Could you check a few things on this model? Use its own coordinates, in mm. A direction names the side the tool comes from. Round coordinates to 2 decimals unless told otherwise and drop trailing zeros. Loops run counter-clockwise (first coordinate to the right, second up) from the corner with the lowest first, then second, coordinate; pieces in that order, holes last. Notation, with made-up numbers: M 15,-28.75 L 58,-28.75 A13 ccw 58,-22.75 Z; hole C 45,88 d3. An arc over 180 degrees is marked long. Answer in a Markdown table with one row per item.
```python
from build123d import *

# Parameters (mm, degrees)
SKETCH1_R           = 14.642304845
BOSS_EXTRUDE1_DEPTH = 2.5
BOSS_EXTRUDE2_DEPTH = 2.5
CUT_EXTRUDE1_REACH  = 22.858
SKETCH3_R           = 2.1
SKETCH4_R           = 4.25
BOSS_EXTRUDE3_DEPTH = 1.75
SKETCH5_R           = 2.6
CUT_EXTRUDE2_DEPTH  = 1.5
CUT_EXTRUDE3_DEPTH  = 22.779730999


with BuildPart() as part:
    # Sketch1 → Boss-Extrude1 (new body)
    with BuildSketch(Plane.XY):
        Circle(SKETCH1_R)
    extrude(amount=BOSS_EXTRUDE1_DEPTH)

    # Sketch2 → Boss-Extrude2 (add)
    with BuildSketch(Plane.XY.offset(2.5)):
        with BuildLine():
            Line((5.5, 7.216878365), (10.563014188, 10.140010969))
            ThreePointArc((10.563014188, 10.140010969), (10.103038739, 10.598381925), (9.623192391, 11.035907729))
            ThreePointArc((9.623192391, 11.035907729), (-0.649210292, 14.627905427), (-10.563014188, 10.140010969))
            Line((-10.563014188, 10.140010969), (-5.5, 7.216878365))
            Line((-5.5, 7.216878365), (-5.5, 3.175426481))
            Line((-5.5, 3.175426481), (-9, 1.154700538))
            Line((-9, 1.154700538), (-14.063014188, 4.077833143))
            ThreePointArc((-14.063014188, 4.077833143), (-12.680607966, -7.321152423), (-3.5, -14.217844112))
            Line((-3.5, -14.217844112), (-3.5, -8.371578903))
            Line((-3.5, -8.371578903), (0, -6.350852961))
            Line((0, -6.350852961), (3.5, -8.371578903))
            Line((3.5, -8.371578903), (3.5, -14.217844112))
            ThreePointArc((3.5, -14.217844112), (12.680607966, -7.321152423), (14.063014188, 4.077833143))
            Line((14.063014188, 4.077833143), (9, 1.154700538))
            Line((9, 1.154700538), (5.5, 3.175426481))
            Line((5.5, 3.175426481), (5.5, 7.216878365))
        make_face()
    extrude(amount=BOSS_EXTRUDE2_DEPTH)

    # Sketch3 → Cut-Extrude1 (cut, up to next)
    with BuildSketch(Plane.XY.offset(2.5), mode=Mode.PRIVATE) as cut_extrude1_sk1:
        with Locations((-9, 5.196152423)):
            Circle(SKETCH3_R)
    cut_extrude1_tool1 = extrude(cut_extrude1_sk1.sketch, amount=-CUT_EXTRUDE1_REACH, mode=Mode.PRIVATE) & part.part
    # Sketch3 → Cut-Extrude1 (cut, up to next)
    with BuildSketch(Plane.XY.offset(2.5), mode=Mode.PRIVATE) as cut_extrude1_sk2:
        with Locations((9, 5.196152423)):
            Circle(SKETCH3_R)
    cut_extrude1_tool2 = extrude(cut_extrude1_sk2.sketch, amount=-CUT_EXTRUDE1_REACH, mode=Mode.PRIVATE) & part.part
    # Sketch3 → Cut-Extrude1 (cut, up to next)
    with BuildSketch(Plane.XY.offset(2.5), mode=Mode.PRIVATE) as cut_extrude1_sk3:
        with Locations((0, -10.392304845)):
            Circle(SKETCH3_R)
    cut_extrude1_tool3 = extrude(cut_extrude1_sk3.sketch, amount=-CUT_EXTRUDE1_REACH, mode=Mode.PRIVATE) & part.part
    add(cut_extrude1_tool1.solids().sort_by_distance((-9, 5.196152, 2.5))[0], mode=Mode.SUBTRACT)
    add(cut_extrude1_tool2.solids().sort_by_distance((9, 5.196152, 2.5))[0], mode=Mode.SUBTRACT)
    add(cut_extrude1_tool3.solids().sort_by_distance((0, -10.392305, 2.5))[0], mode=Mode.SUBTRACT)

    # Sketch4 → Boss-Extrude3 (add)
    with BuildSketch(Plane.XY.offset(5)):
        with Locations(Location((0, 0, 0), (0, 0, 180))):
            Circle(SKETCH4_R)
    extrude(amount=BOSS_EXTRUDE3_DEPTH)

    # Sketch5 → Cut-Extrude2 (cut)
    with BuildSketch(Plane.XY.offset(6.75)):
        Circle(SKETCH5_R)
    extrude(amount=-CUT_EXTRUDE2_DEPTH, mode=Mode.SUBTRACT)

    # Sketch6 → Cut-Extrude3 (cut, through all)
    with BuildSketch(Plane.XY.offset(6.75)):
        with BuildLine():
            Line((2.544199592, -0.535769015), (0.030619782, 2.599819692))
            ThreePointArc((0.030619782, 2.599819692), (-1.626221745, 2.028645567), (-2.544199592, 0.535769015))
            Line((-2.544199592, 0.535769015), (-0.030619782, -2.599819692))
            ThreePointArc((-0.030619782, -2.599819692), (1.626221745, -2.028645567), (2.544199592, -0.535769015))
        make_face()
    extrude(amount=-CUT_EXTRUDE3_DEPTH, mode=Mode.SUBTRACT)


solid = part.part
```
1) I want a section at C-C, the plane y = 6. Please give me the cut outline in (x, z), plus the area to 3 significant figures.
Computed:
| item | result |
|---|---|
| outline | M -13.36,0 L -10.94,0 L -10.94,2.5 L -13.36,2.5 Z; M -7.06,0 L 7.06,0 L 7.06,2.5 L 5.5,2.5 L 5.5,5 L -5.5,5 L -5.5,2.5 L -7.06,2.5 Z; M 10.94,0 L 13.36,0 L 13.36,2.5 L 10.94,2.5 Z |
| area | 74.9 mm² |
2) If we mould it in two halves opening along Y, with no side actions, what happens to faces 1 (the face through (1.73, -7.35, 3.73)), 2 (the face through (2, -12, 2.5)), 3 (the face through (8, 8.66, 3.73))? For each: released by +Y, released by -Y, zero draft, split by the parting line, or undercut.
Computed:
| item | result |
|---|---|
| face 1 | released by -Y |
| face 2 | zero draft |
| face 3 | undercut |
3) I need wall thicknesses on line 1 (Y direction, x = 0, z = 1.6); line 2 (Z direction, x = -7.25, y = -6.5); line 3 (Y direction, x = -1, z = 1.5). Which ranges of each line are inside material? Lowest first, please.
Computed:
| item | result |
|---|---|
| line 1 | y = -14.64 to -12.49, -8.29 to -2.6, 2.6 to 14.64 |
| line 2 | z = 0 to 5 |
| line 3 | y = -14.61 to -12.24, -8.55 to -1.39, 2.4 to 14.61 |
4) I want a section at B-B, the plane z = 3.5. Please give me the cut outline in (x, y).
Computed:
| item | result |
|---|---|
| outline | M -14.06,4.08 A14.64 ccw -3.5,-14.22 L -3.5,-8.37 L 0,-6.35 L 3.5,-8.37 L 3.5,-14.22 A14.64 ccw 14.06,4.08 L 9,1.15 L 5.5,3.18 L 5.5,7.22 L 10.56,10.14 A14.64 ccw -10.56,10.14 L -5.5,7.22 L -5.5,3.18 L -9,1.15 Z; hole M -2.54,0.54 L -0.03,-2.6 A2.6 ccw 2.54,-0.54 L 0.03,2.6 A2.6 ccw Z |
5) I want a section at D-D, the plane y = -9.75. Please give me the cut outline in (x, z), plus the area to 3 significant figures.
Computed:
| item | result |
|---|---|
| outline | M -10.92,0 L -2,0 L -2,2.5 L -3.5,2.5 L -3.5,5 L -10.92,5 Z; M 2,0 L 10.92,0 L 10.92,5 L 3.5,5 L 3.5,2.5 L 2,2.5 Z |
| area | 81.7 mm² |
6) Which directions (+Z, -Z, +X, -X, +Y, -Y) give clear straight access to the entire face, cutting with the end or side of a thin tool? Please do faces 4 (the face through (0, -3, 0)), 5 (the face through (-1.305, -1.01, 2.662)), 6 (the face through (3.5, -11, 4)), 7 (the face through (11, 7, 2.5)).
Computed:
| item | result |
|---|---|
| face 4 | -Z, +X, -X, +Y, -Y |
| face 5 | +Z, -Z |
| face 6 | +Z, -Y |
| face 7 | +Z |
7) Will these pins go through, and if not, where does the flat tip stop? P1, Ø7, axis at x = 9.5, y = 6, coming from the +Z side; P2, Ø1, axis at x = -1.5, y = -2, coming from the +Z side; P3, Ø1.2, axis at y = 4.5, z = 3, coming from the +X side; P4, Ø0.8, axis at y = 5.5, z = 3.5, coming from the -X side.
Computed:
| item | result |
|---|---|
| P1 | stops at z = 5 |
| P2 | stops at z = 6.75 |
| P3 | stops at x = 14.11 |
| P4 | stops at x = -5.5 |
8) I want a section at A-A, the plane y = 0. Please give me the cut outline in (x, z), plus the area to 3 significant figures.
Computed:
| item | result |
|---|---|
| outline | M -14.64,0 L -2.11,0 L -2.11,5.25 L -2.6,5.25 L -2.6,6.75 L -4.25,6.75 L -4.25,5 L -14.64,5 Z; M 2.11,0 L 14.64,0 L 14.64,5 L 4.25,5 L 4.25,6.75 L 2.6,6.75 L 2.6,5.25 L 2.11,5.25 Z |
| area | 131 mm² |
